Geometry check sheet. Reference: the model listing, model coordinates, mm. Give positions to 0.01 mm unless a question says otherwise; leave off trailing zeros. Order: outer loops, then holes, each group sorted by start corner. A loop starts at its lowest first (then second) coordinate and runs counter-clockwise, first axis right, second up. Notation, with made-up numbers: (40.5, 6) - (96.5, 6) arc R30 cw to (96.5, 31) - close; hole circle Ø4 at (15, 17). An arc over 180 degrees is marked (long way). Put each result on its own line as item: value. Start each with the question number.
```python
from build123d import *

# Parameters (mm, degrees)
BOSS_EXTRUDE1_DEPTH = 275.6
CUT_EXTRUDE1_DEPTH  = 342.565498998
CUT_EXTRUDE2_DEPTH  = 342.565498998
CUT_EXTRUDE3_DEPTH  = 587.943701099
CUT_EXTRUDE4_DEPTH  = 587.892777338
FILLET1_R           = 2.75
FILLET2_R           = 0.2


with BuildPart() as part:
    # Sketch1 → Boss-Extrude1 (new, symmetric)
    with BuildSketch(Plane.XY):
        Polygon((0, 0), (201.107183261, -10.856373276), (201.404089876, -5.356373276), (0.296906615, 5.5), align=None)
    extrude(amount=BOSS_EXTRUDE1_DEPTH, both=True)

    # Sketch2 → Cut-Extrude1 (cut, through all)
    with BuildSketch(Plane(origin=(0.296906615, 5.5, 0), x_dir=(0.9985460936510022, -0.053904534636001866, 0), z_dir=(0.053904534636001866, 0.9985460936510022, 0))):
        Polygon((0, 0), (95.4, 275.6), (0, 275.6), align=None)
    extrude(amount=-CUT_EXTRUDE1_DEPTH, mode=Mode.SUBTRACT)

    # Sketch3 → Cut-Extrude2 (cut, through all)
    with BuildSketch(Plane(origin=(0.296906615, 5.5, 0), x_dir=(0.9985460936510022, -0.053904534636001866, 0), z_dir=(0.053904534636001866, 0.9985460936510022, 0))):
        Polygon((0, 0), (95.4, -275.6), (0, -275.6), align=None)
    extrude(amount=-CUT_EXTRUDE2_DEPTH, mode=Mode.SUBTRACT)

    # Sketch4 → Cut-Extrude3 (cut, through all)
    with BuildSketch(Plane.XY.offset(275.6)):
        Polygon((168.751632614, -3.593694993), (201.255636569, -8.106373276), (201.404089876, -5.356373276), align=None)
    extrude(amount=-CUT_EXTRUDE3_DEPTH, mode=Mode.SUBTRACT)

    # Sketch5 → Cut-Extrude4 (cut, through all)
    with BuildSketch(Plane.XY.offset(275.6)):
        Polygon((201.255636569, -8.106373276), (168.454725999, -9.093694993), (201.107183261, -10.856373276), align=None)
    extrude(amount=-CUT_EXTRUDE4_DEPTH, mode=Mode.SUBTRACT)

    # Fillet1
    fillet1_edges = [part.edges().sort_by_distance(p)[0] for p in [
        (47.630648667, -2.571246302, -137.8),
        (47.927555282, 2.928753698, -137.8),
        (47.630648667, -2.571246302, 137.8),
        (47.927555282, 2.928753698, 137.8),
    ]]
    fillet(fillet1_edges, radius=FILLET1_R)

    # Fillet2
    fillet2_edges = [part.edges().sort_by_distance(p)[0] for p in [
        (201.255636569, -8.106373276, 0),
    ]]
    fillet(fillet2_edges, radius=FILLET2_R)


solid = part.part
```
Item 1: Cross-section at B-B (x = 151). Enter the section's corners in (y, z).
Item 2: Thickness scan on line 1 along Y through (x, z) = (168.5, 108); line 2 along Y through (x, z) = (159.5, -2.5). Record the ranges inside material, lowest first.
Item 3: Gauge pin test, flat ends, axial feed: pin 1 Ø2 at (x, z) = (37, -40) entering from -Y; pin 2 Ø1 at (x, z) = (143.5, -181.5) entering from +Y; pin 3 Ø2 at (x, z) = (126.5, -54) entering from -Y. Record the tip position at first contact, or that the pin passes through.
Item 4: Cross-section at A-A (x = 175). Enter the section's corners in (y, z), and give its area (3 significant figures).
Recorded:
1. outline: (-8.15, -275.6) - (-2.64, -275.6) - (-2.64, 275.6) - (-8.15, 275.6) - close
2. line 1: y = -9.09 to -3.58
2. line 2: y = -8.61 to -3.09
3. pin 1: stops at y = -2.05
3. pin 2: stops at y = -2.2
3. pin 3: stops at y = -6.88
4. outline: (-8.9, -275.6) - (-4.46, -275.6) - (-4.46, 275.6) - (-8.9, 275.6) - close
4. area: 2,440 mm^2
